Autodesk Inventor part; units mm, degrees
ref_plane "YZ Plane" through (0, 0, 0) normal (1, 0, 0) x (0, 1, 0)
ref_plane "XZ Plane" through (0, 0, 0) normal (0, 1, 0) x (-1, 0, 0)
ref_plane "XY Plane" through (0, 0, 0) normal (0, 0, 1) x (1, 0, 0)
sketch "Sketch1" plane through (0, 0, 0) normal (0, 0, 1) x (1, 0, 0)
  circle A0 centre (0, 0) radius 13.0482
  circle A1 centre (0, 0) radius 12.0482
  circle A2 centre (0, 0) radius 11.0482
  point P0 (0, 0)
extrude "Extrusion1" add sketch "Sketch1" along normal blind 2 contours A0 | A1
sketch "Sketch2" plane through (0, 0, 2) normal (0, 0, 1) x (1, 0, 0)
  circle A0 centre (0, 0) radius 13.0482
  circle A1 centre (0, 0) radius 13.0482
extrude "Extrusion2" add sketch "Sketch2" along normal blind 2
sketch "Sketch3" plane through (0, 0, 4) normal (0, 0, 1) x (1, 0, 0)
  circle A0 centre (0, 0) radius 13.0482
  circle A1 centre (0, 0) radius 2.15
  dimension "d4" = 4.3
extrude "Extrusion3" cut sketch "Sketch3" against normal through all contours A1
properties part number "EndCap"
Geometry check sheet. Reference: the model listing, model coordinates, mm. A direction names the side the tool comes from. Round coordinates to 2 decimals unless told otherwise and drop trailing zeros. Loops run counter-clockwise (first coordinate to the right, second up) from the corner with the lowest first, then second, coordinate; pieces in that order, holes last. Notation, with made-up numbers: (40.25, 4.25) -> (90.25, 4.25) arc R18 cw to (90.25, 14.25) -> close; hole circle Ø10 at (22.25, 73.25). An arc over 180 degrees is marked (long way). Use a Markdown table: item, result.
(1) Mould release check, pull along X, two halves, no side actions. Record for faces 3 (the cylindrical face through (-10.355, 7.94, 1.972)), 4 (the flat face through (-11, 3, 0)), 5 (the cylindrical face through (-2.15, 0.09, 3.01)): released by +X, released by -X, zero draft, split by the parting line, or undercut.
Calculated:
| item | result |
|---|---|
| face 3 | split by the parting line |
| face 4 | zero draft |
| face 5 | undercut |
(2) Go/stop test with flat-tipped pins: P1, Ø1, axis at y = -2, z = 3, coming from the -X side; P2, Ø1, axis at x = -4, z = 0.5, coming from the +Y side; P3, Ø4, axis at x = 0, y = 0, coming from the -Z side; P4, Ø1.5, axis at x = 7, z = 1.5, coming from the -Y side. Record where each tip stops, or that it passes through.
Calculated:
| item | result |
|---|---|
| P1 | x = -12.96 |
| P2 | y = 12.57 |
| P3 | through |
| P4 | y = -11.45 |
(3) Scan lines: probe 1 along Y at (x, z) = (0, 1.6); probe 2 along Y at (x, z) = (0, 3.6); probe 3 along Z at (x, y) = (-7.25, -3.5). Record each from-to range of solid material in increasing order.
Calculated:
| item | result |
|---|---|
| probe 1 | -13.05 to -11.05, 11.05 to 13.05 |
| probe 2 | -13.05 to -2.15, 2.15 to 13.05 |
| probe 3 | 2 to 4 |
(4) Sectioned sample at D-D (y = 8). Enter the section's corners in (x, z), then the cut area to 3 significant figures.
Calculated:
| item | result |
|---|---|
| outline | (-10.31, 0) -> (-7.62, 0) -> (-7.62, 2) -> (7.62, 2) -> (7.62, 0) -> (10.31, 0) -> (10.31, 4) -> (-10.31, 4) -> close |
| area | 52.0 mm² |
(5) Sectioned sample at C-C (z = 3.45). Enter the section's corners in (x, y).
Calculated:
| item | result |
|---|---|
| outline | circle Ø26.1 at (0, 0); hole circle Ø4.3 at (0, 0) |
(6) Sectioned sample at A-A (y = 0). Enter the section's corners in (x, z).
Calculated:
| item | result |
|---|---|
| outline | (-13.05, 0) -> (-11.05, 0) -> (-11.05, 2) -> (-2.15, 2) -> (-2.15, 4) -> (-13.05, 4) -> close; (2.15, 2) -> (11.05, 2) -> (11.05, 0) -> (13.05, 0) -> (13.05, 4) -> (2.15, 4) -> close |
(7) Set-up check for faces 1 (the flat face through (2.3, 0.2, 2)), 2 (the flat face through (0, -3, 4)): record each of +Z, -Z, +X, -X, +Y, -Y from which the full face is reachable in a straight line by a thin tool's end or side.
Calculated:
| item | result |
|---|---|
| face 1 | -Z |
| face 2 | +Z, +X, -X, +Y, -Y |
